```python
from build123d import *

# Parameters (mm, degrees)
SKETCH1_W               = 99
SKETCH1_H               = 25
SKETCH1_W_2             = 93
SKETCH1_H_2             = 19
BOSS_EXTRUDE1_DEPTH     = 10
SKETCH2_R               = 40
CUT_EXTRUDE1_DEPTH      = 8
SKETCH5_W               = 10
SKETCH5_H               = 25
BOSS_EXTRUDE5_DEPTH     = 2
SKETCH6_W               = 6
SKETCH6_H               = 19
BOSS_EXTRUDE6_DEPTH     = 2
SKETCH7_W               = 8
SKETCH7_H               = 3
BOSS_EXTRUDE7_DEPTH     = 30
FILLET5_R               = 3
FILLET7_R               = 5
FILLET8_R               = 20
FILLET9_R               = 1.5
FILLET10_R              = 6
FILLET11_R              = 3
SKETCH8_W               = 20
SKETCH8_H               = 25
BOSS_EXTRUDE8_DEPTH     = 2
SKETCH9_W               = 9.8
SKETCH9_H               = 12
BOSS_EXTRUDE9_DEPTH     = 10
SKETCH10_R              = 2
CUT_EXTRUDE2_DEPTH      = 23
FILLET12_R              = 6
CUT_EXTRUDE5_DEPTH      = 65.857536204
CUT_EXTRUDE5_DEPTH_BACK = 65.857536204
SKETCH12_W              = 9.8
SKETCH12_H              = 12
FILLET13_R              = 2


with BuildPart() as part:
    # Sketch1 → Boss-Extrude1 (new body)
    with BuildSketch(Plane(origin=(0, 0, 0), x_dir=(1, 0, 0), z_dir=(0, 1, 0))):
        Rectangle(SKETCH1_W, SKETCH1_H)
        Rectangle(SKETCH1_W_2, SKETCH1_H_2, mode=Mode.SUBTRACT)
    extrude(amount=BOSS_EXTRUDE1_DEPTH)

    # Sketch2 → Cut-Extrude1 (cut)
    with BuildSketch(Plane.XY.offset(12.5)):
        with Locations((21.780912994, 42.853113242)):
            Circle(SKETCH2_R)
    extrude(amount=-CUT_EXTRUDE1_DEPTH, mode=Mode.SUBTRACT)

    # Sketch5 → Boss-Extrude5 (add)
    with BuildSketch(Plane.XZ):
        with Locations((-29.5, 0)):
            Rectangle(SKETCH5_W, SKETCH5_H)
    extrude(amount=-BOSS_EXTRUDE5_DEPTH)

    # Sketch6 → Boss-Extrude6 (add)
    with BuildSketch(Plane.XZ):
        with Locations((43.5, 0)):
            Rectangle(SKETCH6_W, SKETCH6_H)
    extrude(amount=-BOSS_EXTRUDE6_DEPTH)

    # Sketch7 → Boss-Extrude7 (add)
    with BuildSketch(Plane(origin=(0, 10, 0), x_dir=(1, 0, 0), z_dir=(0, 1, 0))):
        with Locations((-32.5, -11)):
            Rectangle(SKETCH7_W, SKETCH7_H)
    extrude(amount=BOSS_EXTRUDE7_DEPTH)

    # Fillet5
    fillet5_edges = [part.edges().sort_by_distance(p)[0] for p in [
        (-34.5, 1, 9.5),
        (-24.5, 1, 9.5),
        (-24.5, 1, -9.5),
        (-34.5, 1, -9.5),
        (40.5, 1, -9.5),
        (40.5, 1, 9.5),
    ]]
    fillet(fillet5_edges, radius=FILLET5_R)

    # Fillet7
    fillet7_edges = [part.edges().sort_by_distance(p)[0] for p in [
        (44.599172136, 10, 11),
    ]]
    fillet(fillet7_edges, radius=FILLET7_R)

    # Fillet8
    fillet8_edges = [part.edges().sort_by_distance(p)[0] for p in [
        (-1.037346149, 10, 11),
    ]]
    fillet(fillet8_edges, radius=FILLET8_R)

    # Fillet9
    fillet9_edges = [part.edges().sort_by_distance(p)[0] for p in [
        (46.5, 6, 9.5),
        (46.5, 6, -9.5),
        (-46.5, 5, -9.5),
        (-46.5, 5, 9.5),
        (-49.5, 5, 12.5),
        (-49.5, 5, -12.5),
        (49.5, 5, -12.5),
        (49.5, 5, 12.5),
    ]]
    fillet(fillet9_edges, radius=FILLET9_R)

    # Fillet10
    fillet10_edges = [part.edges().sort_by_distance(p)[0] for p in [
        (-36.5, 10, 11),
        (-28.5, 10, 11),
    ]]
    fillet(fillet10_edges, radius=FILLET10_R)

    # Fillet11
    fillet11_edges = [part.edges().sort_by_distance(p)[0] for p in [
        (-36.5, 40, 11),
        (-28.5, 40, 11),
    ]]
    fillet(fillet11_edges, radius=FILLET11_R)

    # Sketch8 → Boss-Extrude8 (add)
    with BuildSketch(Plane.XZ):
        Rectangle(SKETCH8_W, SKETCH8_H)
    extrude(amount=-BOSS_EXTRUDE8_DEPTH)

    # Sketch9 → Boss-Extrude9 (add)
    with BuildSketch(Plane.XZ):
        Rectangle(SKETCH9_W, SKETCH9_H)
    extrude(amount=BOSS_EXTRUDE9_DEPTH)

    # Sketch10 → Cut-Extrude2 (cut)
    with BuildSketch(Plane(origin=(4.9, 0, 0), x_dir=(0, 0, -1), z_dir=(1, 0, 0))):
        with Locations((0, -5)):
            Circle(SKETCH10_R)
    extrude(amount=-CUT_EXTRUDE2_DEPTH, mode=Mode.SUBTRACT)

    # Fillet12
    fillet12_edges = [part.edges().sort_by_distance(p)[0] for p in [
        (0, -10, 6),
        (0, -10, -6),
    ]]
    fillet(fillet12_edges, radius=FILLET12_R - 0.0001)  # a hair under: the kernel refuses the full size

    # Sketch12 → Cut-Extrude5 (cut, two sides: drawn at the far end of the back side and taken through both)
    with BuildSketch(Plane.XZ.offset(-CUT_EXTRUDE5_DEPTH_BACK)):
        Rectangle(SKETCH12_W, SKETCH12_H)
    extrude(amount=CUT_EXTRUDE5_DEPTH + CUT_EXTRUDE5_DEPTH_BACK, mode=Mode.SUBTRACT)

    # Fillet13
    fillet13_edges = [part.edges().sort_by_distance(p)[0] for p in [
        (-10, 1, 9.5),
        (10, 1, 9.5),
        (10, 1, -9.5),
        (-10, 1, -9.5),
    ]]
    fillet(fillet13_edges, radius=FILLET13_R)


solid = part.part
```
Geometry: final body of the model. Coordinates: model frame, mm. A direction names the side the tool comes from. Coordinates: 2 decimals unless noted, no trailing zeros. Loops run counter-clockwise (first coordinate to the right, second up) from the corner with the lowest first, then second, coordinate; pieces in that order, holes last. Notation, with made-up numbers: (76.25, -12) -> (86.25, -12) arc R23 cw to (86.25, -2) -> close; hole circle Ø1 at (19.25, -24.5). An arc over 180 degrees is marked (long way). Use a Markdown table: item, result. Add a question column.
(1) Line query: line 1 along Z through (x, y) = (-4, 6.5); line 2 along X through (y, z) = (5.5, 8); line 3 along Y through (x, z) = (-34, -10). Output: solid intervals per line, ascending.
(2) Section query A-A, the plane z = -4. Return loops of the section in (x, y), plus the area to 3 significant figures.
(3) Pin query (flat end, axial travel): pin 1 Ø10 at (x, z) = (42.5, -1.5) entering from +Y; pin 2 Ø1.5 at (y, z) = (14, 7.5) entering from +X; pin 3 Ø1.5 at (y, z) = (29.5, 11) entering from -X; pin 4 Ø2.5 at (y, z) = (28.5, 10.5) entering from +X. Return the tip coordinate at first contact, or that it passes through.
(4) Section query D-D, the plane x = 33. Return loops of the section in (y, z), plus the area to 3 significant figures.
(5) Mould query, pull axis X, two halves, no side actions, for faces 1 (the flat face through (-46.5, 5, 0)), 2 (the cylindrical face through (-29.36, 39.1, 10.98)), 3 (the flat face through (-14, 8, 12.5)). Classes: pulls with the +X half, pulls with the -X half, needs draft (parallel to the pull), parting line crosses it, or undercut.
(6) Section query B-B, the plane x = 18.5. Return loops of the section in (y, z).
(7) Section query C-C, the plane y = 36. Return loops of the section in (x, z).
(8) Access query for faces 4 (the flat face through (-24.5, 1, 0)), 5 (the flat face through (-15, 10, 11)), 6 (the flat face through (-1, 5, -9.5)), 7 (the cylindrical face through (-38.211, 11.804, 10.979)), 8 (the flat face through (-49.5, 5, 0)). Directions: +Z, -Z, +X, -X, +Y, -Y. A direction counts if a zero-diameter tool reaches every point of the face in a straight line with its end or side. Return the directions, or none.
Answer:
| question | item | result |
|---|---|---|
| 1 | line 1 | z = -12.5 to -9.5, 9.5 to 12.5 |
| 1 | line 2 | x = -49.5 to -46.5, 46.5 to 49.5 |
| 1 | line 3 | y = 0 to 10 |
| 2 | outline | (-49.5, 0) -> (-46.5, 0) -> (-46.5, 10) -> (-49.5, 10) -> close; (-34.5, 0) -> (-24.5, 0) -> (-24.5, 2) -> (-34.5, 2) -> close; (-10, 0) -> (-4.9, 0) -> (-4.9, 2) -> (-10, 2) -> close; (4.9, 0) -> (10, 0) -> (10, 2) -> (4.9, 2) -> close; (40.5, 0) -> (49.5, 0) -> (49.5, 10) -> (46.5, 10) -> (46.5, 2) -> (40.5, 2) -> close |
| 2 | area | 112 mm^2 |
| 3 | pin 1 | stops at y = 10 |
| 3 | pin 2 | passes through |
| 3 | pin 3 | stops at x = -36.5 |
| 3 | pin 4 | stops at x = -28.5 |
| 4 | outline | (0, -12.5) -> (10, -12.5) -> (10, -9.5) -> (0, -9.5) -> close; (0, 9.5) -> (4.46, 9.5) -> (4.46, 12.5) -> (0, 12.5) -> close |
| 4 | area | 43.4 mm^2 |
| 5 | face 1 | undercut |
| 5 | face 2 | pulls with the +X half |
| 5 | face 3 | needs draft |
| 6 | outline | (0, -12.5) -> (10, -12.5) -> (10, -9.5) -> (0, -9.5) -> close; (0, 9.5) -> (2.99, 9.5) -> (2.99, 12.5) -> (0, 12.5) -> close |
| 7 | outline | (-36.5, 9.5) -> (-28.5, 9.5) -> (-28.5, 12.5) -> (-36.5, 12.5) -> close |
| 8 | face 4 | +Y, -Y |
| 8 | face 5 | +Z, -Z, +X, +Y |
| 8 | face 6 | +Y |
| 8 | face 7 | +Z, -Z, -X, +Y |
| 8 | face 8 | +Z, -Z, -X, +Y, -Y |
